from build123d import *

# Parameters (mm, degrees)
SKETCH_1_W          = 10
SKETCH_1_H          = 150
EXTRUDE_1_DEPTH     = 10
SKETCH_3_W          = 10
SKETCH_3_H          = 10
CUT_EXTRUDE_1_DEPTH = 5
HOLE_WIZARD_M4_1_D  = 3.3
SKETCH_7_R          = 2.868052952
SKETCH_7_R_2        = 4
CUT_EXTRUDE_2_DEPTH = 1


with BuildPart() as part:
    # 草图1 → 凸台-拉伸1 (new body)
    with BuildSketch(Plane.XY):
        with Locations((5, -75)):
            Rectangle(SKETCH_1_W, SKETCH_1_H)
    extrude(amount=EXTRUDE_1_DEPTH)

    # 草图3 → 切除-拉伸1 (cut)
    with BuildSketch(Plane(origin=(0, 0, 0), x_dir=(-1, 0, 0), z_dir=(0, 0, -1))):
        with Locations((-5, -5)):
            Rectangle(SKETCH_3_W, SKETCH_3_H)
        with Locations((-5, -145)):
            Rectangle(SKETCH_3_W, SKETCH_3_H)
    extrude(amount=-CUT_EXTRUDE_1_DEPTH, mode=Mode.SUBTRACT)

    # M4 螺纹孔1 (through all)
    with Locations(Plane.XY.offset(10)):
        with Locations((5, -5), (5, -145)):
            Hole(HOLE_WIZARD_M4_1_D / 2)

    # 草图7 → 切除-拉伸2 (cut)
    with BuildSketch(Plane.XY.offset(10)):
        with Locations((5, -5)):
            Circle(SKETCH_7_R)
        with Locations((5, -145)):
            Circle(SKETCH_7_R_2)
    extrude(amount=-CUT_EXTRUDE_2_DEPTH, mode=Mode.SUBTRACT)


solid = part.part
For this review, take the finished solid that the model builds, in its own axes (mm). A direction names the side the tool comes from. Coordinates: 2 decimals unless noted, no trailing zeros. Order: outer loops, then holes, each group sorted by start corner. A loop starts at its lowest first (then second) coordinate and runs counter-clockwise, first axis right, second up. Notation, with made-up numbers: (-16.5, 55.25) - (8.5, 55.25) arc R27 cw to (8.5, 93.25) - close; hole circle Ø3 at (5.25, 80.5). An arc over 180 degrees is marked (long way). Answer as CSV lines item,"result". Start each with the question number.
1) Machinability: for faces 1 (the cylindrical face through (2.724, -6.745, 9.507)), 2 (the flat face through (5, -10, 2)), 3 (the flat face through (7, -145, 5)), which of the approach directions +Z, -Z, +X, -X, +Y, -Y give a long, thin tool a straight path to every point of the face, cutting with its end or side? Answer none if there is none.
2) Draft analysis for pull direction X (two halves, no side actions). For faces 4 (the flat face through (5, -140, 2)), 5 (the flat face through (0, -76, 5)), 6 (the cylindrical face through (4.239, -146.464, 6.972)), state which applies: +X half, -X half, draft (parallel to the pull), parting line (faces both ways), or undercut.
3) Add section A-A (y = -145). State the section outline as (x, z) points.
4) To check wall thickness, follow line 1 along Y through (x, z) = (5, 9.2); line 2 along Y through (x, z) = (5, 5.9); line 3 along Y through (x, z) = (6.25, 1.75). State the ranges of each line that lie inside material, in increasing order. Write a range as [from, to].
5) Insertion check: P1, Ø3, axis at x = 6.5, y = -146, coming from the -Z side; P2, Ø2.5, axis at x = 4.5, y = -147, coming from the +Z side; P3, Ø5.5, axis at x = 4, z = 2, coming from the +Y side. Each pin has a flat end and moves straight along its axis. Give the tip position at first contact, or say it passes through.
6) Add section B-B (x = 5). State the section outline as (y, z) points, then the cut area to 3 significant figures.
7) Add section C-C (y = -5). State the section outline as (x, z) points.
Result:
1,face 1,"+Z"
1,face 2,"-Z, +X, -X, +Y"
1,face 3,"-Z, +X, -X, -Y"
2,face 4,"draft"
2,face 5,"-X half"
2,face 6,"undercut"
3,outline,"(0, 5) - (3.35, 5) - (3.35, 9) - (1, 9) - (1, 10) - (0, 10) - close; (6.65, 5) - (10, 5) - (10, 10) - (9, 10) - (9, 9) - (6.65, 9) - close"
4,line 1,"[-150, -149], [-141, -7.87], [-2.13, 0]"
4,line 2,"[-150, -146.65], [-143.35, -6.65], [-3.35, 0]"
4,line 3,"[-140, -10]"
5,P1,"z = 5"
5,P2,"z = 9"
5,P3,"y = -10"
6,outline,"(-150, 5) - (-146.65, 5) - (-146.65, 9) - (-149, 9) - (-149, 10) - (-150, 10) - close; (-143.35, 5) - (-140, 5) - (-140, 0) - (-10, 0) - (-10, 5) - (-6.65, 5) - (-6.65, 9) - (-7.87, 9) - (-7.87, 10) - (-141, 10) - (-141, 9) - (-143.35, 9) - close; (-3.35, 5) - (0, 5) - (0, 10) - (-2.13, 10) - (-2.13, 9) - (-3.35, 9) - close"
6,area,"1,360 mm^2"
7,outline,"(0, 5) - (3.35, 5) - (3.35, 9) - (2.13, 9) - (2.13, 10) - (0, 10) - close; (6.65, 5) - (10, 5) - (10, 10) - (7.87, 10) - (7.87, 9) - (6.65, 9) - close"
